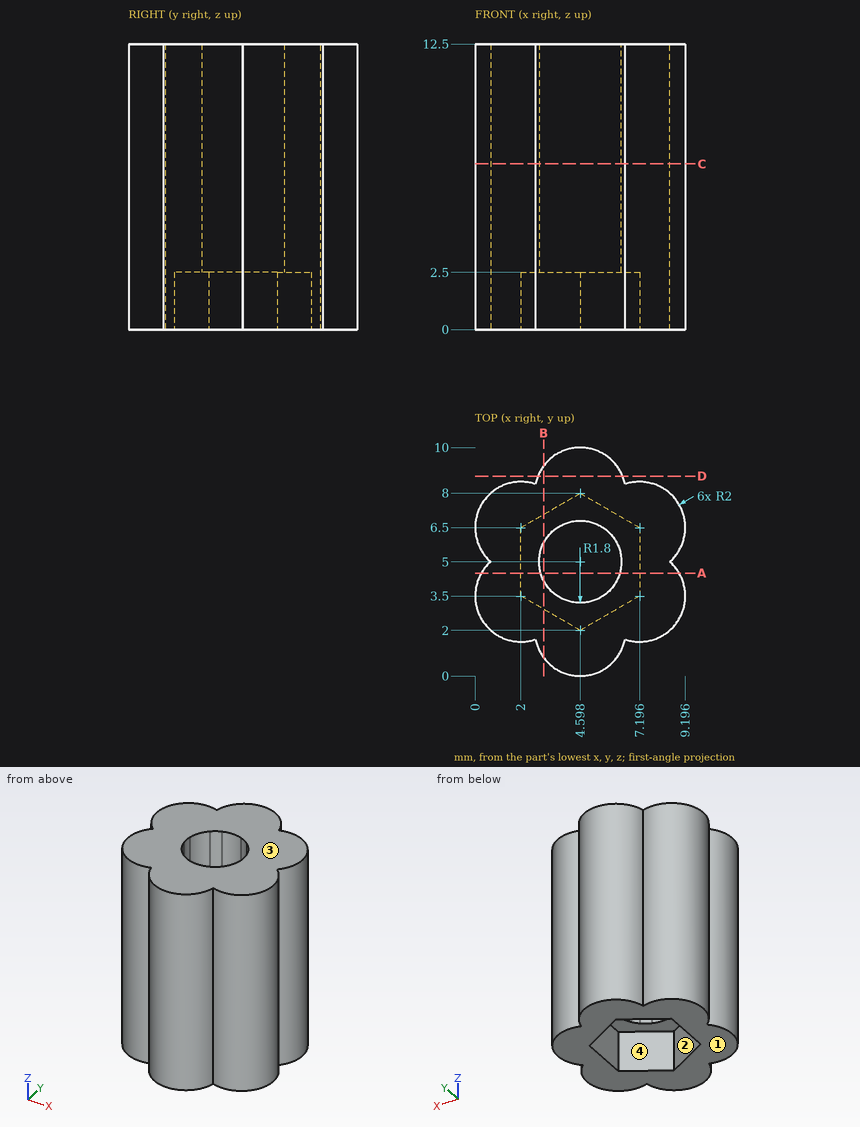
Job drawing, mm, ordinate dimensions from the low corner. One solid piece. A direction names the side the tool comes from. Round coordinates to 2 decimals unless told otherwise and drop trailing zeros. Write each loop counter-clockwise with the first axis right and the second up, starting at its lowest first coordinate (ties: lowest second). Pieces come first, ordered by that corner, then holes. Notation, with made-up numbers: M 42.25,27 L 66.25,27 A23 cw 66.25,36 Z; hole C -12,52 d4. An arc over 180 degrees is marked long. Return JSON: item names as keys, results as strings. Group by question number.
(1) Pin check, flat tips, straight feed: pin 1 Ø1 at (y, z) = (5, 9) entering from -X; pin 2 Ø0.8 at (y, z) = (5.5, 2) entering from -X; pin 3 Ø2.5 at (x, y) = (3.5, 5) entering from -Z. Stop position of each tip, or through.
(2) Saw through at C-C on z = 7.25. Write the cut outline in (x, y).
(3) Two-plate mould, pull along X, no slides. Class the marked faces 1 and 2: +X half, -X half, draft (parallel to the pull), parting line (faces both ways), or undercut.
(4) Saw through at A-A on y = 4.5. Write the cut outline in (x, z).
(5) Which spindle directions (+Z, -Z, +X, -X, +Y, -Y) get a long thin tool onto all of the face, cutting with end or side? Do the marked faces 3 and 4. Say none if no direction does.
(6) Drill centre lines: probe 1 along Y at (x, z) = (4.5, 9); probe 2 along Z at (x, y) = (3, 3.75); probe 3 along X at (y, z) = (6, 10.5) (1 decimal). Where is each one in solid material? Low to high.
(7) Saw through at D-D on y = 8.75. Write the cut outline in (x, z).
(8) Saw through at B-B on x = 3. Write the cut outline in (y, z), then the cut area to 3 significant figures.
Returned:
{
 "1": {"pin 1": "x = 0.27", "pin 2": "x = 0.09", "pin 3": "z = 2.5"},
 "2": {"outline": "M 0.68,5 A2 ccw 2.64,1.6 A2 ccw 6.56,1.6 A2 ccw 8.52,5 A2 ccw 6.56,8.4 A2 ccw 2.64,8.4 A2 ccw Z; hole C 4.6,5 d3.6"},
 "3": {"face 1": "draft", "face 2": "undercut"},
 "4": {"outline": "M 0.27,0 L 2,0 L 2,2.5 L 2.87,2.5 L 2.87,12.5 L 0.27,12.5 Z; M 6.33,2.5 L 7.2,2.5 L 7.2,0 L 8.93,0 L 8.93,12.5 L 6.33,12.5 Z"},
 "5": {"face 3": "+Z, +X, -X, +Y, -Y", "face 4": "-Z"},
 "6": {"probe 1": "0 to 3.2, 6.8 to 10", "probe 2": "2.5 to 12.5", "probe 3": "0.1 to 3.1, 6.1 to 9.1"},
 "7": {"outline": "M 2.74,0 L 6.45,0 L 6.45,12.5 L 2.74,12.5 Z"},
 "8": {"outline": "M 0.8,0 L 2.92,0 L 2.92,2.5 L 4.17,2.5 L 4.17,12.5 L 0.8,12.5 Z; M 5.83,2.5 L 7.08,2.5 L 7.08,0 L 9.2,0 L 9.2,12.5 L 5.83,12.5 Z", "area": "78.1 mm²"}
}
